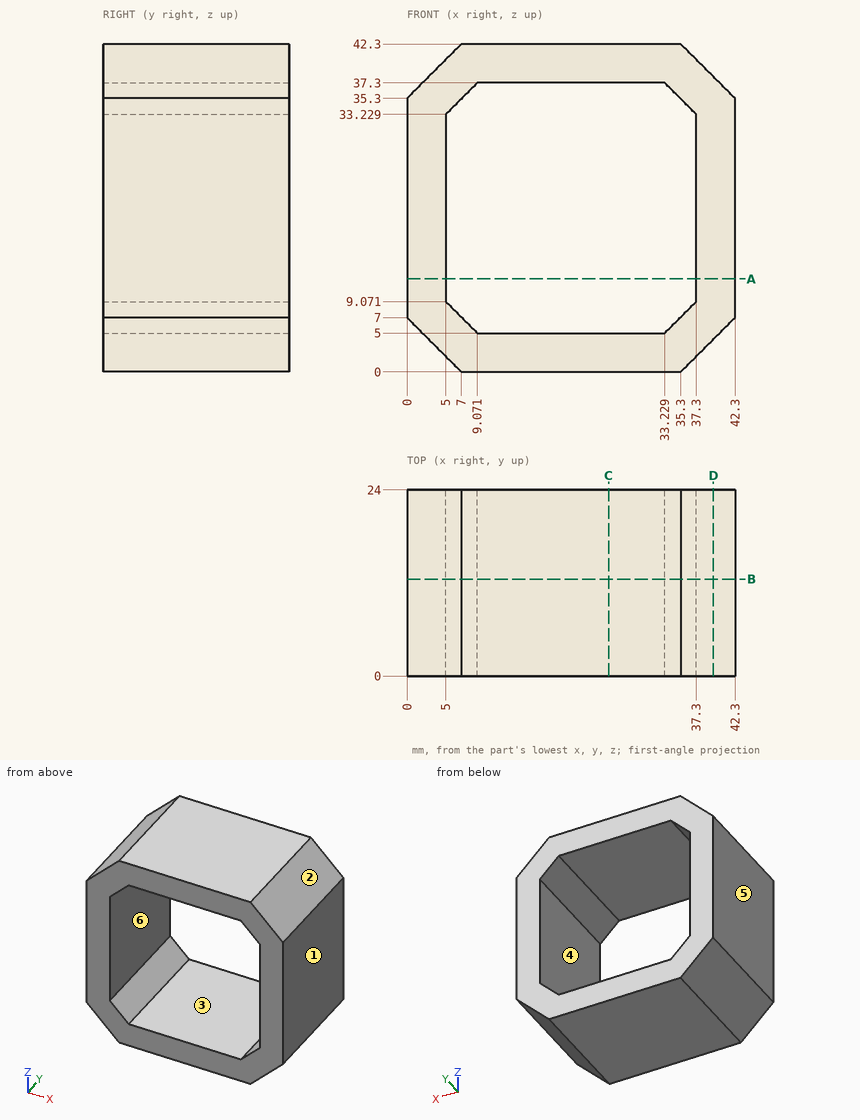
Check sheet for the drawn part. Datum: minimum x, y, z corner. Units: mm. A direction names the side the tool comes from. Round coordinates to 2 decimals unless told otherwise and drop trailing zeros. Order: outer loops, then holes, each group sorted by start corner. A loop starts at its lowest first (then second) coordinate and runs counter-clockwise, first axis right, second up.
1) Section check A-A (z = 12). Record the boundary of the cut face in (x, y).
2) Scan lines: line 1 (Z direction, x = 10, y = 6.5); line 2 (Z direction, x = 6.5, y = 11). Record each from-to range of solid material in increasing order.
3) Mould release check, pull along Z, two halves, no side actions. Record for the marked faces 1, 2, 3 and 4: +Z half, -Z half, draft (parallel to the pull), parting line (faces both ways), or undercut.
4) Section check B-B (y = 12.5). Record the boundary of the cut face in (x, z).
5) Tool access check on the marked faces 5 and 6. Record the directions out of +Z, -Z, +X, -X, +Y, -Y that give a thin tool (end or side, any length) a straight path to the whole face; none if there is none.
6) Section check C-C (x = 26). Record the boundary of the cut face in (y, z).
7) Section check D-D (x = 39.5). Record the boundary of the cut face in (y, z).
8) Go/stop test with a flat-tipped pin: pin 1 Ø2 at (y, z) = (7, 36.5) entering from -X. Record where the tip stops, or that it passes through.
Result:
1. outline: (0, 0) - (5, 0) - (5, 24) - (0, 24) - close; (37.3, 0) - (42.3, 0) - (42.3, 24) - (37.3, 24) - close
2. line 1: z = 0 to 5, 37.3 to 42.3
2. line 2: z = 0.5 to 7.57, 34.73 to 41.8
3. face 1: draft
3. face 2: +Z half
3. face 3: undercut
3. face 4: undercut
4. outline: (0, 7) - (7, 0) - (35.3, 0) - (42.3, 7) - (42.3, 35.3) - (35.3, 42.3) - (7, 42.3) - (0, 35.3) - close; hole (5, 9.07) - (9.07, 5) - (33.23, 5) - (37.3, 9.07) - (37.3, 33.23) - (33.23, 37.3) - (9.07, 37.3) - (5, 33.23) - close
5. face 5: +Z, -Z, -X, +Y, -Y
5. face 6: +Y, -Y
6. outline: (0, 0) - (24, 0) - (24, 5) - (0, 5) - close; (0, 37.3) - (24, 37.3) - (24, 42.3) - (0, 42.3) - close
7. outline: (0, 4.2) - (24, 4.2) - (24, 38.1) - (0, 38.1) - close
8. pin 1: stops at x = 0.2
